Here's how the part is built. I have some questions about the finished solid (model axes, mm). Face numbers are marked on the shaded views. A direction names the side the tool comes from. Round coordinates to 2 decimals unless told otherwise and drop trailing zeros. Write each loop counter-clockwise with the first axis right and the second up, starting at its lowest first coordinate (ties: lowest second). Pieces come first, ordered by that corner, then holes. Notation, with made-up numbers: M -21.5,-7 L 17.5,-7 A13 cw 17.5,0 Z; hole C 41.5,36 d4. An arc over 180 degrees is marked long. Use one line per item in the form item = value. Start each with the question number.
Q1. I want a section at D-D on z = 235. List the corners of the cut face in (x, y) for me, and give its area (3 significant figures).
Q2. I'm going to push flat-ended pins straight in: pin 1 Ø15 at (x, z) = (23.5, -6) entering from -Y; pin 2 Ø5 at (x, z) = (39, 167) entering from -Y; pin 3 Ø3 at (x, z) = (28.5, 107.5) entering from +Y; pin 4 Ø10.5 at (x, y) = (62.58, 0.5) entering from +Z. Where does each tip first touch, or does it pass through?
Q3. We'd pull the mould along Z, two halves only. Please class the marked faces 1 and 2: +Z half, -Z half, draft (parallel to the pull), parting line (faces both ways), or undercut.
Q4. I want a section at B-B on z = 110. List the corners of the cut face in (x, y) for me.
Q5. For the marked faces 3 and 4, which set-ups out of +Z, -Z, +X, -X, +Y, -Y let a thin tool reach every point of the face, with its end or its side?
Q6. I want a section at A-A on z = -10. List the corners of the cut face in (x, y) for me, and give its area (3 significant figures).
Q7. I need wall thicknesses on line 1 along Z through (x, y) = (18.5, -10.5); line 2 along Y through (x, z) = (24, 58); line 3 along Z through (x, y) = (47.5, -0.5). Which ranges of each line are inside material? Lowest first, please. Write a range as from..to.
Q8. I want a section at C-C on x = 48. List the corners of the cut face in (y, z) for me, and give its area (3 significant figures).
```python
from build123d import *

# Parameters (mm, degrees)
F0_R      = 4
F1_DEPTH  = 5
F2_R      = 5.5
F2_R_2    = 4
F3_DEPTH  = 25
F4_DEPTH  = 10
F5_W      = 30
F5_H      = 5
F6_DEPTH  = 25
F7_R      = 4
F8_DEPTH  = 7
F9_R      = 9.5
F9_R_2    = 4
F10_DEPTH = 15
F11_R     = 8
F11_R_2   = 4
F12_DEPTH = 75
F13_R     = 9.5
F14_DEPTH = 15
F15_R     = 8
F16_DEPTH = 15
F17_R     = 6.5
F18_DEPTH = 240
F20_W     = 20
F20_H     = 21
F21_DEPTH = 10
F23_R     = 15
F24_DEPTH = 12.5
F25_R     = 5
F26_DEPTH = 70
F27_R     = 6
F28_DEPTH = 25
F30_W     = 40
F30_H     = 20
F31_DEPTH = 10
F32_W     = 10
F32_H     = 20
F33_DEPTH = 20
F34_R     = 5
F35_DEPTH = 20


with BuildPart() as f1:
    # F0 (on Top) → F1 (new body)
    with BuildSketch(Plane.XY):
        Polygon((72.578296, 13.000988), (-27.421704, 13.000988), (-27.421704, -11.999012), (7.578296, -11.999012), (7.578296, -21.999012), (37.578296, -21.999012), (37.578296, -11.999012), (72.578296, -11.999012), align=None)
        with Locations((-17.421704, 0.500988)):
            Circle(F0_R, mode=Mode.SUBTRACT)
        with Locations((22.578296, 0.500988)):
            Circle(F0_R, mode=Mode.SUBTRACT)
        with Locations((62.578296, 0.500988)):
            Circle(F0_R, mode=Mode.SUBTRACT)
    extrude(amount=F1_DEPTH)

    # F2 (on face) → F3 (join)
    with BuildSketch(Plane.XY.offset(5)):
        with Locations((-17.421704, 0.500988)):
            Circle(F2_R)
        with Locations((-17.421704, 0.500988)):
            Circle(F2_R_2, mode=Mode.SUBTRACT)
        with Locations((62.578296, 0.500988)):
            Circle(F2_R)
        with Locations((62.578296, 0.500988)):
            Circle(F2_R_2, mode=Mode.SUBTRACT)
    extrude(amount=F3_DEPTH)

    # F2 (on face) → F4 (join)
    with BuildSketch(Plane.XY.offset(5)):
        with Locations((-17.421704, 0.500988)):
            Circle(F2_R)
        with Locations((-17.421704, 0.500988)):
            Circle(F2_R_2, mode=Mode.SUBTRACT)
        with Locations((62.578296, 0.500988)):
            Circle(F2_R)
        with Locations((62.578296, 0.500988)):
            Circle(F2_R_2, mode=Mode.SUBTRACT)
    extrude(amount=-F4_DEPTH)

    # F5 (on face) → F6 (join)
    with BuildSketch(Plane(origin=(0, 0, 0), x_dir=(1, 0, 0), z_dir=(0, 0, -1))):
        with Locations((22.578296, 19.499012)):
            Rectangle(F5_W, F5_H)
    extrude(amount=F6_DEPTH)

    # F7 (on face) → F8 (join)
    with BuildSketch(Plane.XY.offset(5)):
        Polygon((12.578296, 6.274491), (12.578296, -5.272514), (22.578296, -11.046017), (32.578296, -5.272514), (32.578296, 6.274491), (22.578296, 12.047994), align=None)
        with Locations((22.578296, 0.500988)):
            Circle(F7_R, mode=Mode.SUBTRACT)
    extrude(amount=F8_DEPTH)

    # F9 (on face) → F10 (join)
    with BuildSketch(Plane.XY.offset(12)):
        with Locations((22.578296, 0.500988)):
            Circle(F9_R)
        with Locations((22.578296, 0.500988)):
            Circle(F9_R_2, mode=Mode.SUBTRACT)
    extrude(amount=F10_DEPTH)

    # F11 (on face) → F12 (join)
    with BuildSketch(Plane.XY.offset(27)):
        with Locations((22.578296, 0.500988)):
            Circle(F11_R)
        with Locations((22.578296, 0.500988)):
            Circle(F11_R_2, mode=Mode.SUBTRACT)
    extrude(amount=F12_DEPTH)

    # F13 (on face) → F14 (join)
    with BuildSketch(Plane.XY.offset(102)):
        with Locations((22.578296, 0.500988)):
            Circle(F13_R)
    extrude(amount=F14_DEPTH)

    # F15 (on face) → F16 (join)
    with BuildSketch(Plane.XY.offset(117)):
        with Locations((22.578296, 0.500988)):
            Circle(F15_R)
    extrude(amount=F16_DEPTH)

    # F17 (on face) → F18 (join)
    with BuildSketch(Plane.XY.offset(5)):
        with Locations((44.578296, 0)):
            Circle(F17_R)
    extrude(amount=F18_DEPTH)

    # F20 (on offset) → F21 (join, symmetric)
    with BuildSketch(Plane.XY.offset(110)):
        with Locations((44.578296, -0.499012)):
            Rectangle(F20_W, F20_H)
    extrude(amount=F21_DEPTH, both=True)

    # F23 (on offset) → F24 (join, symmetric)
    with BuildSketch(Plane.YZ.offset(45)):
        with Locations((0, 235)):
            Circle(F23_R)
    extrude(amount=F24_DEPTH, both=True)

    # F25 (on face) → F26 (join)
    with BuildSketch(Plane(origin=(32.5, 0, 0), x_dir=(0, -1, 0), z_dir=(-1, 0, 0))):
        with Locations((0, 235)):
            Circle(F25_R)
    extrude(amount=-F26_DEPTH)

    # F27 (on face) → F28 (cut)
    with BuildSketch(Plane.XZ.offset(21.999012)):
        with Locations((22.578296, -10)):
            Circle(F27_R)
    extrude(amount=-F28_DEPTH, mode=Mode.SUBTRACT)

    # F30 (on face) → F31 (join)
    with BuildSketch(Plane.XZ.offset(10.999012)):
        with Locations((44.578296, 110)):
            Rectangle(F30_W, F30_H)
    extrude(amount=F31_DEPTH)

    # F32 (on face) → F33 (join)
    with BuildSketch(Plane.XZ.offset(20.999012)):
        with Locations((59.578296, 110)):
            Rectangle(F32_W, F32_H)
        with Locations((29.578296, 110)):
            Rectangle(F32_W, F32_H)
    extrude(amount=F33_DEPTH)

    # F34 (on face) → F35 (join, through all)
    with BuildSketch(Plane(origin=(54.578296, 0, 0), x_dir=(0, -1, 0), z_dir=(-1, 0, 0))):
        with Locations((30.999012, 110)):
            Circle(F34_R)
    extrude(amount=F35_DEPTH)


solid = f1.part
```
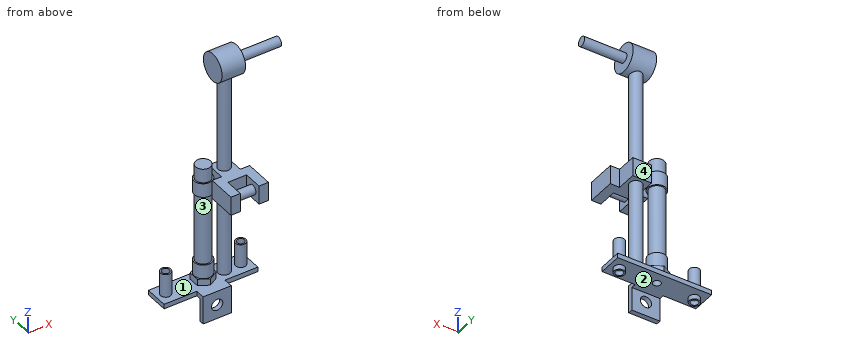
Reported:
q1.outline = M 32.5,-15 L 57.5,-15 L 57.5,-5 L 102.5,-5 L 102.5,5 L 57.5,5 L 57.5,15 L 32.5,15 Z
q1.area = 1,200 mm^2
q2.pin_1 = -22
q2.pin_2 = -5.72
q2.pin_3 = 8.91
q2.pin_4 = 250
q3.face_1 = undercut
q3.face_2 = -Z half
q4.outline = C 22.58,0.5 d19; M 24.58,-41 L 34.58,-41 L 34.58,-36 L 54.58,-36 L 54.58,-41 L 64.58,-41 L 64.58,-11 L 54.58,-11 L 54.58,10 L 34.58,10 L 34.58,-11 L 24.58,-11 Z; hole M 34.58,-26 L 54.58,-26 L 54.58,-21 L 34.58,-21 Z
q5.face_3 = none
q5.face_4 = +X, -X, +Y
q6.outline = M 7.58,-22 L 16.58,-22 L 16.58,-17 L 7.58,-17 Z; M 28.58,-22 L 37.58,-22 L 37.58,-17 L 28.58,-17 Z
q6.area = 90.0 mm^2
q7.line_1 = 0..5
q7.line_2 = -7.37..-3.24, 4.24..8.37
q7.line_3 = 0..249.99
q8.outline = C -31,110 d10; M -21,100 L -5.53,100 L -5.53,5 L -12,5 L -12,0 L 13,0 L 13,5 L 5.53,5 L 5.53,100 L 10,100 L 10,120 L 5.53,120 L 5.53,221.06 A15 ccw long -5.53,221.06 L -5.53,120 L -21,120 Z
q8.area = 3,690 mm^2
